Build history of the part. All positions in model axes, mm. A direction names the side the tool comes from. Give positions to 0.01 mm unless a question says otherwise; leave off trailing zeros. Loops run counter-clockwise (first coordinate to the right, second up) from the corner with the lowest first, then second, coordinate; pieces in that order, holes last. Notation, with made-up numbers: (67.25, -39) -> (123.25, -39) arc R17 cw to (123.25, -15) -> close; hole circle Ø4 at (85.25, 73.25). An arc over 180 degrees is marked (long way). Answer as a JSON object with one key per item and string values. Group by question number.
from build123d import *

# Parameters (mm, degrees)
SKETCH_1_R                   = 15
EXTRUDE_1_DEPTH              = 3
SKETCH_2_R                   = 6
EXTRUDE_2_DEPTH              = 7
HOLE_WIZARD_M3_1_D           = 3.4
HOLE_WIZARD_M3_1_DEPTH       = 14.54
HOLE_WIZARD_M3_1_CSINK_D     = 6.72
HOLE_WIZARD_M3_1_CSINK_ANGLE = 118
HOLE_WIZARD_M3_1_TIP         = 1.021463052
SKETCH_6_R                   = 7
SKETCH_6_R_2                 = 6
EXTRUDE_3_DEPTH              = 2


with BuildPart() as part:
    # 草图1 → 凸台-拉伸1 (new body)
    with BuildSketch(Plane.XY):
        Circle(SKETCH_1_R)
    extrude(amount=EXTRUDE_1_DEPTH)

    # 草图2 → 凸台-拉伸2 (add)
    with BuildSketch(Plane.XY.offset(3)):
        Circle(SKETCH_2_R)
    extrude(amount=EXTRUDE_2_DEPTH)

    # M3 六角凹锥坑螺钉的锥形沉头孔1
    with Locations(Plane(origin=(0, 11, 3), x_dir=(1, 0, 0), z_dir=(0, 0, 1))):
        with Locations((0, 0), (-9.526279442, -16.5), (9.526279442, -16.5)):
            CounterSinkHole(HOLE_WIZARD_M3_1_D / 2, HOLE_WIZARD_M3_1_CSINK_D / 2, depth=HOLE_WIZARD_M3_1_DEPTH, counter_sink_angle=HOLE_WIZARD_M3_1_CSINK_ANGLE)
            with Locations((0, 0, -(HOLE_WIZARD_M3_1_DEPTH + HOLE_WIZARD_M3_1_TIP / 2))):  # 118° drill point
                Cone(0, HOLE_WIZARD_M3_1_D / 2, HOLE_WIZARD_M3_1_TIP, mode=Mode.SUBTRACT)

    # 草图6 → 凸台-拉伸3 (add)
    with BuildSketch(Plane.XY.offset(3)):
        Circle(SKETCH_6_R)
        Circle(SKETCH_6_R_2, mode=Mode.SUBTRACT)
    extrude(amount=EXTRUDE_3_DEPTH)


solid = part.part
(1) Saw through at D-D on z = 3.75. List the corners of the cut face in (x, y), plus the area to 3 significant figures.
(2) Probe line 1 along Y through (x, z) = (0, 0.75); line 2 along X through (y, z) = (-5.5, 1.2); line 3 along Z through (x, y) = (-1.5, -7.5). List the from-to ranges inside material, lowest first. Write a range as [from, to].
(3) Saw through at B-B on x = 0. List the corners of the cut face in (y, z).
(4) Saw through at C-C on y = 0. List the corners of the cut face in (x, z).
(5) Saw through at A-A on y = -5.5. List the corners of the cut face in (x, z), plus the area to 3 significant figures.
(6) 3-axis set-ups, long thin cutter, end or side, ignore diameter. For faces 4 (the cylindrical face through (11.225, -5.425, 0.987)), 5 (the flat face through (6, 2, 5)): which of +Z, -Z, +X, -X, +Y, -Y reach the whole face in a straight line?
(7) Pin check, flat tips, straight feed: pin 1 (15 mm diameter, centred on x = 6.5, y = 2.5, fed in from +Z); pin 2 (4.5 mm diameter, centred on x = -9.53, y = -5.5, fed in from +Z); pin 3 (2 mm diameter, centred on x = 4, z = 7.5, fed in from -Y); pin 4 (2.5 mm diameter, centred on x = 0, y = 11, fed in from +Z). Stop position of each tip, or through.
(8) Pull direction X, two halves, no side cores. Call faces 1 (the cylindrical face through (-11.097, -6.151, 0.987)), 2 (the flat face through (0, 0, 10)), 3 (the cylindrical face through (6.466, -2.681, 3.986)): pulls with the +X half, pulls with the -X half, needs draft (parallel to the pull), parting line crosses it, or undercut.
Calculated:
{
 "1": {"outline": "circle Ø14 at (0, 0)", "area": "154 mm^2"},
 "2": {"line 1": "y = [-15, 9.3], [12.7, 15]", "line 2": "x = [-13.96, -11.23], [-7.83, 7.83], [11.23, 13.96]", "line 3": "z = [0, 3]"},
 "3": {"outline": "(-15, 0) -> (9.3, 0) -> (9.3, 2) -> (7.64, 3) -> (7, 3) -> (7, 5) -> (6, 5) -> (6, 10) -> (-6, 10) -> (-6, 5) -> (-7, 5) -> (-7, 3) -> (-15, 3) -> close; (12.7, 0) -> (15, 0) -> (15, 3) -> (14.36, 3) -> (12.7, 2) -> close"},
 "4": {"outline": "(-15, 0) -> (15, 0) -> (15, 3) -> (7, 3) -> (7, 5) -> (6, 5) -> (6, 10) -> (-6, 10) -> (-6, 5) -> (-7, 5) -> (-7, 3) -> (-15, 3) -> close"},
 "5": {"outline": "(-13.96, 0) -> (-11.23, 0) -> (-11.23, 2) -> (-12.89, 3) -> (-13.96, 3) -> close; (-7.83, 0) -> (7.83, 0) -> (7.83, 2) -> (6.17, 3) -> (4.33, 3) -> (4.33, 5) -> (2.4, 5) -> (2.4, 10) -> (-2.4, 10) -> (-2.4, 5) -> (-4.33, 5) -> (-4.33, 3) -> (-6.17, 3) -> (-7.83, 2) -> close; (11.23, 0) -> (13.96, 0) -> (13.96, 3) -> (12.89, 3) -> (11.23, 2) -> close", "area": "101 mm^2"},
 "6": {"face 4": "+Z, -Z", "face 5": "+Z"},
 "7": {"pin 1": "stops at z = 10", "pin 2": "stops at z = 2.34", "pin 3": "stops at y = -5.2", "pin 4": "passes through"},
 "8": {"face 1": "undercut", "face 2": "needs draft", "face 3": "parting line crosses it"}
}
